For this review, use the dimensioned drawing (mm, ordinates from the lowest corner) and the shaded views. Coordinates: 2 decimals unless noted, no trailing zeros. Loops run counter-clockwise (first coordinate to the right, second up) from the corner with the lowest first, then second, coordinate; pieces in that order, holes last. Notation, with made-up numbers: (1.25, -3) -> (55.25, -3) arc R20 ccw to (55.25, 9) -> close; hole circle Ø4 at (69.25, 80). An arc over 180 degrees is marked (long way). Use one line per item in the form item = value. Start each with the question number.
1. Consider section B-B (z = 29). State the section outline as (x, y) points.
2. Consider section A-A (y = 2.05). State how many separate pieces and enclosed holes the cut face has, then the cut area to 3 significant figures.
3. Consider section D-D (x = 11). State the section outline as (y, z) points.
4. Consider section C-C (z = 5). State the section outline as (x, y) points, then the cut area to 3 significant figures.
5. Wall thickness on line 1 (X direction, y = 1.8, z = 33); line 2 (X direction, y = 1.15, z = 4); line 3 (X direction, y = 1.95, z = 32.5): over which ranges is each line inside the solid? List them lowest first. Write a range as from..to.
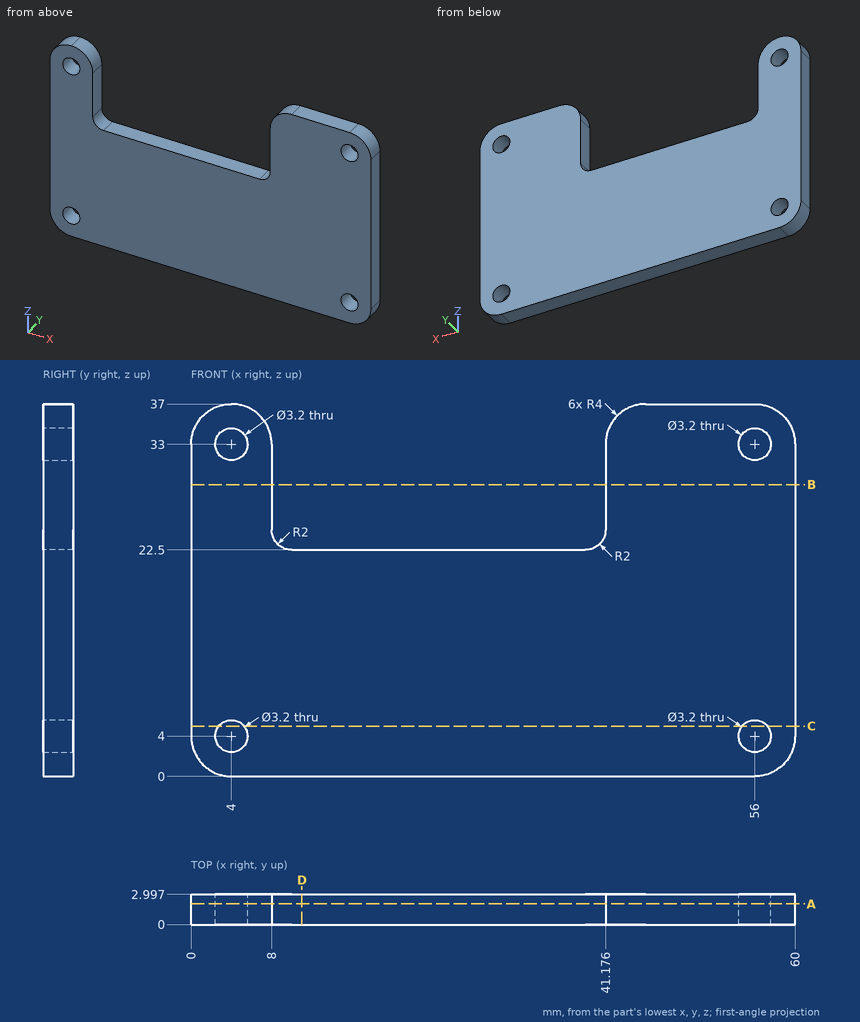
Geometry check:
q1.outline = (0, 0) -> (8, 0) -> (8, 3) -> (0, 3) -> close; (41.18, 0) -> (60, 0) -> (60, 3) -> (41.18, 3) -> close
q2.separate_pieces = 1
q2.enclosed_holes = 4
q2.area = 1,690 mm²
q3.outline = (0, 0) -> (3, 0) -> (3, 22.5) -> (0, 22.5) -> close
q4.outline = (0, 0) -> (2.75, 0) -> (2.75, 3) -> (0, 3) -> close; (5.25, 0) -> (54.75, 0) -> (54.75, 3) -> (5.25, 3) -> close; (57.25, 0) -> (60, 0) -> (60, 3) -> (57.25, 3) -> close
q4.area = 165 mm²
q5.line_1 = 0..2.4, 5.6..8, 41.18..54.4, 57.6..60
q5.line_2 = 0..2.4, 5.6..54.4, 57.6..60
q5.line_3 = 0..2.48, 5.52..8, 41.18..54.48, 57.52..60
